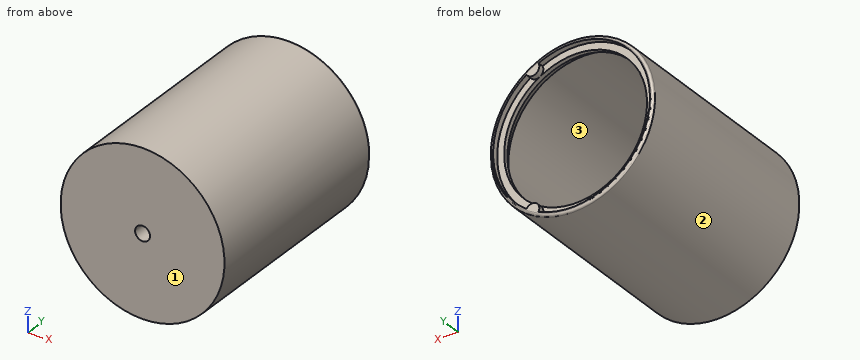
```python
from build123d import *

# Parameters (mm, degrees)
ESQUISSE1_R             = 35.25
BOSS_EXTRU_1_DEPTH      = 90
CONG_1_R                = 1
ESQUISSE4_R             = 33.75
ENL_V_MAT_EXTRU_3_DEPTH = 2.5
ESQUISSE5_R             = 32.75
ENL_V_MAT_EXTRU_4_DEPTH = 84
ESQUISSE6_R             = 33.75
ESQUISSE6_R_2           = 30.75
BOSS_EXTRU_2_DEPTH      = 10
CHANFREIN1_SIZE         = 8
CHANFREIN1_SIZE_2       = 4.618802154
BOSS_EXTRU_3_START      = 2.5
BOSS_EXTRU_3_DEPTH      = 2.5
ESQUISSE8_R             = 6.2
BOSS_EXTRU_4_DEPTH      = 8
ESQUISSE2_R             = 3.2
ENL_V_MAT_EXTRU_1_DEPTH = 103.884036697
CONG_2_R                = 1.5


with BuildPart() as part:
    # Esquisse1 → Boss.-Extru.1 (new body)
    with BuildSketch(Plane(origin=(0, 0, 0), x_dir=(1, 0, 0), z_dir=(0, 1, 0))):
        with Locations(Location((0, 0, 0), (0, 0, 90))):
            Circle(ESQUISSE1_R)
    extrude(amount=BOSS_EXTRU_1_DEPTH)

    # Congé1
    cong_1_edges = [part.edges().sort_by_distance(p)[0] for p in [
        (0, 90, 35.25),
    ]]
    fillet(cong_1_edges, radius=CONG_1_R)

    # Esquisse4 → Enlèv. mat.-Extru.3 (cut)
    with BuildSketch(Plane(origin=(0, 90, 0), x_dir=(1, 0, 0), z_dir=(0, 1, 0))):
        with Locations(Location((0, 0, 0), (0, 0, 270))):
            Circle(ESQUISSE4_R)
    extrude(amount=-ENL_V_MAT_EXTRU_3_DEPTH, mode=Mode.SUBTRACT)

    # Esquisse5 → Enlèv. mat.-Extru.4 (cut)
    with BuildSketch(Plane(origin=(0, 87.5, 0), x_dir=(1, 0, 0), z_dir=(0, 1, 0))):
        with Locations(Location((0, 0, 0), (0, 0, 270))):
            Circle(ESQUISSE5_R)
    extrude(amount=-ENL_V_MAT_EXTRU_4_DEPTH, mode=Mode.SUBTRACT)

    # Esquisse6 → Boss.-Extru.2 (add)
    with BuildSketch(Plane(origin=(0, 87.5, 0), x_dir=(1, 0, 0), z_dir=(0, 1, 0))):
        with Locations(Location((0, 0, 0), (0, 0, 270))):
            Circle(ESQUISSE6_R)
        with Locations(Location((0, 0, 0), (0, 0, 270))):
            Circle(ESQUISSE6_R_2, mode=Mode.SUBTRACT)
    extrude(amount=-BOSS_EXTRU_2_DEPTH)

    # Chanfrein1
    # the kernel refuses this chamfer: 8, 4.618802154 mm, written as the material it takes off along each edge
    with BuildSketch(Plane(origin=(0, 77.5, 0), x_dir=(0, 0, 1), z_dir=(-1, 0, 0))) as chanfrein1_piece_1_section:
        Polygon((30.75, CHANFREIN1_SIZE), (30.75 + CHANFREIN1_SIZE_2, 0), (30.75, 0), align=None)
    chanfrein1_piece_1 = revolve(axis=Axis((0, 77.5, 0), (0, 1, 0)), mode=Mode.PRIVATE)
    chanfrein1_piece_1 = chanfrein1_piece_1 & Plane(origin=(0, 83.835682002, 0), x_dir=(0, 0, 1), z_dir=(0, 1, 0)) * Cylinder(32.75, 142, mode=Mode.PRIVATE)
    add(chanfrein1_piece_1, mode=Mode.SUBTRACT)

    # Esquisse7 → Boss.-Extru.3 (add)
    with BuildSketch(Plane(origin=(0, 87.5, 0), x_dir=(1, 0, 0), z_dir=(0, 1, 0)).offset(BOSS_EXTRU_3_START)):
        with BuildLine():
            ThreePointArc((14.212824392, 30.61140511), (15.375, 26.630281166), (19.403842275, 27.614369538))
            ThreePointArc((19.403842275, 27.614369538), (16.875, 29.228357378), (14.212824392, 30.61140511))
        make_face()
        with BuildLine():
            ThreePointArc((14.212824392, -30.61140511), (16.875, -29.228357378), (19.403842275, -27.614369538))
            ThreePointArc((19.403842275, -27.614369538), (15.375, -26.630281166), (14.212824392, -30.61140511))
        make_face()
    extrude(amount=-BOSS_EXTRU_3_DEPTH)

    # Esquisse8 → Boss.-Extru.4 (add)
    with BuildSketch(Plane(origin=(0, 3.5, 0), x_dir=(1, 0, 0), z_dir=(0, 1, 0))):
        with Locations(Location((0, 0, 0), (0, 0, 270))):
            Circle(ESQUISSE8_R)
    extrude(amount=BOSS_EXTRU_4_DEPTH)

    # Esquisse2 → Enlèv. mat.-Extru.1 (cut, through all)
    with BuildSketch(Plane.XZ):
        with Locations(Location((0, 0, 0), (0, 0, 270))):
            Circle(ESQUISSE2_R)
    extrude(amount=-ENL_V_MAT_EXTRU_1_DEPTH, mode=Mode.SUBTRACT)

    # Congé2
    cong_2_edges = [part.edges().sort_by_distance(p)[0] for p in [
        (0, 3.5, -32.75),
        (0, 3.5, -6.2),
        (0, 11.5, -6.2),
    ]]
    fillet(cong_2_edges, radius=CONG_2_R)


solid = part.part
```
CAD build for the part. Positions are in the model's coordinates, mm. Face numbers are marked on the shaded views. Give positions to 0.01 mm unless a question says otherwise; leave off trailing zeros. Order: outer loops, then holes, each group sorted by start corner. A loop starts at its lowest first (then second) coordinate and runs counter-clockwise, first axis right, second up.
(1) Drill centre lines: L1, parallel to X at y = 6, z = 0; L2, parallel to X at y = 88, z = 0; L3, parallel to X at y = 86.8, z = 0. Where is each one in solid material? Low to high.
(2) Mould opens along X. For the marked faces 1, 2 and 3 say: released by +X, released by -X, zero draft, split by the parting line, or undercut.
(3) Flat gauge pins, fed straight in: pin 1 (12 mm diameter, centred on x = 15, z = -6, fed in from +Y); pin 2 (2 mm diameter, centred on y = 69, z = 26, fed in from +X); pin 3 (20 mm diameter, centred on x = 21.5, z = -11, fed in from +Y); pin 4 (12 mm diameter, centred on x = -5.5, z = -4, fed in from +Y). Where does each tip first touch, or does it go through?
(4) Saw through at C-C, the plane y = 45. Give the cut face in (x, z), then the cut area to 3 significant figures.
Results found:
1. L1: x = -35.25 to -32.75, -6.2 to -3.2, 3.2 to 6.2, 32.75 to 35.25
1. L2: x = -35.25 to -33.75, 33.75 to 35.25
1. L3: x = -35.25 to -30.75, 30.75 to 35.25
2. face 1: zero draft
2. face 2: split by the parting line
2. face 3: undercut
3. pin 1: stops at y = 3.5
3. pin 2: stops at x = 24.85
3. pin 3: stops at y = 90
3. pin 4: stops at y = 11.5
4. outline: circle Ø70.5 at (0, 0); hole circle Ø65.5 at (0, 0)
4. area: 534 mm2
